from build123d import *

# Parameters (mm, degrees)
SKETCH_1_R                 = 225
EXTRUDE_1_DEPTH            = 50
SKETCH_2_R                 = 25
CUT_EXTRUDE_1_DEPTH        = 334.541601603
SKETCH_3_R                 = 175
SKETCH_3_R_2               = 75
CUT_EXTRUDE_3_DEPTH        = 20
CUT_EXTRUDE_3_DRAFT        = -30
MIRROR_1_COPY_1_SKETCH_R   = 175
MIRROR_1_COPY_1_SKETCH_R_2 = 75
MIRROR_1_COPY_1_DEPTH      = 20
MIRROR_1_COPY_1_DRAFT      = -30
CHAMFER_1_SIZE             = 5
SKETCH_4_R                 = 25.852351377
CUT_EXTRUDE_4_DEPTH        = 329.10059433


with BuildPart() as part:
    # 草图1 → 凸台-拉伸1 (new, symmetric)
    with BuildSketch(Plane.XY):
        Circle(SKETCH_1_R)
    extrude(amount=EXTRUDE_1_DEPTH, both=True)

    # 草图2 → 切除-拉伸1 (cut, through all)
    with BuildSketch(Plane.XY.offset(50)):
        Circle(SKETCH_2_R)
    extrude(amount=-CUT_EXTRUDE_1_DEPTH, mode=Mode.SUBTRACT)


with BuildPart() as cut_extrude_3_tool:
    # 草图3 → 切除-拉伸3 (with draft: the straight prism first)
    with BuildSketch(Plane.XY.offset(50)):
        Circle(SKETCH_3_R)
        Circle(SKETCH_3_R_2, mode=Mode.SUBTRACT)
    extrude(amount=-CUT_EXTRUDE_3_DEPTH)
    # 切除-拉伸3: the draft: its side faces are tilted about the plane it starts from
    cut_extrude_3_sides = [cut_extrude_3_tool.faces().sort_by_distance(p)[0] for p in [
        (-175, 0, 40),
        (-75, 0, 40),
    ]]
    draft(cut_extrude_3_sides, Plane.XY.offset(50), CUT_EXTRUDE_3_DRAFT)


with BuildPart() as part_1:
    add(part.part)

    # 切除-拉伸3: cut by cut_extrude_3_tool
    add(cut_extrude_3_tool.part, mode=Mode.SUBTRACT)


with BuildPart() as mirror_1_copy_1_tool:
    # 镜向1 copy 1 sketch → 镜向1 copy 1 (with draft: the straight prism first)
    with BuildSketch(Plane(origin=(0, 0, -50), x_dir=(1, 0, 0), z_dir=(0, 0, -1))):
        Circle(MIRROR_1_COPY_1_SKETCH_R)
        Circle(MIRROR_1_COPY_1_SKETCH_R_2, mode=Mode.SUBTRACT)
    extrude(amount=-MIRROR_1_COPY_1_DEPTH)
    # 镜向1 copy 1: the draft: its side faces are tilted about the plane it starts from
    mirror_1_copy_1_sides = [mirror_1_copy_1_tool.faces().sort_by_distance(p)[0] for p in [
        (-175, 0, -40),
        (-75, 0, -40),
    ]]
    draft(mirror_1_copy_1_sides, Plane(origin=(0, 0, -50), x_dir=(1, 0, 0), z_dir=(0, 0, -1)), MIRROR_1_COPY_1_DRAFT)


with BuildPart() as part_2:
    add(part_1.part)

    # 镜向1 copy 1: cut by mirror_1_copy_1_tool
    add(mirror_1_copy_1_tool.part, mode=Mode.SUBTRACT)

    # 倒角1
    chamfer_1_edges = [part_2.edges().sort_by_distance(p)[0] for p in [
        (-225, 0, -50),
        (-225, 0, 50),
    ]]
    chamfer(chamfer_1_edges, length=CHAMFER_1_SIZE)

    # 草图4 → 切除-拉伸4 (cut, through all)
    with BuildSketch(Plane.XY.offset(30)):
        with Locations((0, 124.095015256)):
            Circle(SKETCH_4_R)
    extrude(amount=-CUT_EXTRUDE_4_DEPTH, mode=Mode.SUBTRACT)


solid = part_2.part
Geometry check sheet. Reference: the model listing, model coordinates, mm. A direction names the side the tool comes from. Coordinates: 2 decimals unless noted, no trailing zeros. Order: outer loops, then holes, each group sorted by start corner. A loop starts at its lowest first (then second) coordinate and runs counter-clockwise, first axis right, second up. Notation, with made-up numbers: (20, -39.5) - (60, -39.5) arc R24 cw to (60, -27.5) - close; hole circle Ø7 at (6.25, -37.75). An arc over 180 degrees is marked (long way). Answer in a Markdown table with one row per item. Add a question column.
1) Release check for a two-part mould opening along X. For faces 4 (the conical face through (156.594, -49.314, -31.251)), 5 (the flat face through (-18, 18, -50)), 6 (the cylindrical face through (-224.782, 9.893, 0.63)) record: +X half, -X half, draft (parallel to the pull), parting line (faces both ways), or undercut.
2) Gauge pin test, flat ends, axial feed: P1, Ø5, axis at y = -169.5, z = 11, coming from the +X side; P2, Ø4, axis at y = -111, z = 14.5, coming from the -X side; P3, Ø10, axis at y = 99, z = 13, coming from the -X side. Record the tip position at first contact, or that the pin passes through.
3) Cross-section at A-A, the plane y = 0. Record the cut outline in (x, z).
4) Cross-section at B-B, the plane x = 0. State how many separate pieces and enclosed holes the cut face has, then the cut area to 3 significant figures.
5) Set-up check for faces 1 (the flat face through (70, 70, -30)), 2 (the flat face through (70, -70, 30)), 3 (the cylindrical face through (23.846, 7.509, 0.7)): record each of +Z, -Z, +X, -X, +Y, -Y from which the full face is reachable in a straight line by a thin tool's end or side.
6) Material ranges on line 1 along Y through (x, z) = (0, 29); line 2 along X through (y, z) = (-39.5, -35); line 3 along Y through (x, z) = (-47, 30.5), recorded low to high. Write a range as [from, to].
7) Cross-section at C-C, the plane z = 36.5. Record the cut outline in (x, y), then the cut area to 3 significant figures.
Check result:
| question | item | result |
|---|---|---|
| 1 | face 4 | undercut |
| 1 | face 5 | draft |
| 1 | face 6 | parting line |
| 2 | P1 | stops at x = 150.78 |
| 2 | P2 | stops at x = -196.83 |
| 2 | P3 | stops at x = -204.42 |
| 3 | outline | (-225, -45) - (-220, -50) - (-175, -50) - (-163.45, -30) - (-86.55, -30) - (-75, -50) - (-25, -50) - (-25, 50) - (-75, 50) - (-86.55, 30) - (-163.45, 30) - (-175, 50) - (-220, 50) - (-225, 45) - close; (25, -50) - (75, -50) - (86.55, -30) - (163.45, -30) - (175, -50) - (220, -50) - (225, -45) - (225, 45) - (220, 50) - (175, 50) - (163.45, 30) - (86.55, 30) - (75, 50) - (25, 50) - close |
| 4 | separate pieces | 3 |
| 4 | enclosed holes | 0 |
| 4 | area | 29,800 mm² |
| 5 | face 1 | -Z |
| 5 | face 2 | +Z |
| 5 | face 3 | +Z, -Z |
| 6 | line 1 | y = [-225, -25], [25, 98.24], [149.95, 225] |
| 6 | line 2 | x = [-221.51, -161.58], [-73.75, 73.75], [161.58, 221.51] |
| 6 | line 3 | y = [-220.04, -156.85], [-72.33, 72.33], [156.85, 220.04] |
| 7 | outline | circle Ø450 at (0, 0); circle Ø165.59 at (0, 0); hole circle Ø334.41 at (0, 0); hole circle Ø50 at (0, 0) |
| 7 | area | 90,800 mm² |
